from build123d import *

# Parameters (mm, degrees)
SKETCH1_R           = 12.5
BOSS_EXTRUDE1_DEPTH = 3.175
SKETCH2_R           = 42
BOSS_EXTRUDE2_DEPTH = 1
SKETCH3_R           = 40
BOSS_EXTRUDE3_DEPTH = 10


with BuildPart() as part:
    # Sketch1 → Boss-Extrude1 (new body)
    with BuildSketch(Plane.XY):
        Circle(SKETCH1_R)
    extrude(amount=-BOSS_EXTRUDE1_DEPTH)

    # Sketch2 → Boss-Extrude2 (add)
    with BuildSketch(Plane.XY):
        Circle(SKETCH2_R)
    extrude(amount=BOSS_EXTRUDE2_DEPTH)

    # Sketch3 → Boss-Extrude3 (add)
    with BuildSketch(Plane.XY.offset(1)):
        Circle(SKETCH3_R)
    extrude(amount=BOSS_EXTRUDE3_DEPTH)


solid = part.part
Check sheet for the modelled part. Datum: model origin and axes. Units: mm. A direction names the side the tool comes from. Round coordinates to 2 decimals unless told otherwise and drop trailing zeros. Order: outer loops, then holes, each group sorted by start corner. A loop starts at its lowest first (then second) coordinate and runs counter-clockwise, first axis right, second up.
Q1. Scan lines: L1, parallel to Z at x = -16, y = 37.5; L2, parallel to Z at x = 10.5, y = 35; L3, parallel to Y at x = -19, z = 7.25. Record each from-to range of solid material in increasing order.
Filled sheet:
L1: z = 0 to 1
L2: z = 0 to 11
L3: y = -35.2 to 35.2
Q2. Set-up check for faces 1 (the face through (40.06, 12.62, 0.49)), 2 (the face through (11.923, 3.755, -1.565)), 3 (the face through (-8.67, -39.05, 5.93)): record each of +Z, -Z, +X, -X, +Y, -Y from which the full face is reachable in a straight line by a thin tool's end or side.
Filled sheet:
face 1: +Z, -Z
face 2: -Z
face 3: +Z
Q3. Cross-section at D-D, the plane y = -31. Enter the section's corners in (x, z), plus the area to 3 significant figures.
Filled sheet:
outline: (-28.34, 0) - (28.34, 0) - (28.34, 1) - (25.28, 1) - (25.28, 11) - (-25.28, 11) - (-25.28, 1) - (-28.34, 1) - close
area: 562 mm2
Q4. Cross-section at C-C, the plane z = 6. Enter the section's corners in (x, y), plus the area to 3 significant figures.
Filled sheet:
outline: circle Ø80 at (0, 0)
area: 5,030 mm2
Q5. Cross-section at A-A, the plane y = 0. Enter the section's corners in (x, z) (3 decimals).
Filled sheet:
outline: (-42, 0) - (-12.5, 0) - (-12.5, -3.175) - (12.5, -3.175) - (12.5, 0) - (42, 0) - (42, 1) - (40, 1) - (40, 11) - (-40, 11) - (-40, 1) - (-42, 1) - close
Q6. Depth check by flat-ended pin: P1, Ø5, axis at y = -3.5, z = 6, coming from the +X side; P2, Ø3, axis at x = 32.5, z = 0, coming from the +Y side; P3, Ø1, axis at x = -18.5, z = 0.5, coming from the -Y side. Enter the tip coordinate at first touch or a pass-through.
Filled sheet:
P1: stops at x = 39.99
P2: stops at y = 28.34
P3: stops at y = -37.95
